Autodesk Inventor part; units mm, degrees
ref_plane "YZ Plane" through (0, 0, 0) normal (1, 0, 0) x (0, 1, 0)
ref_plane "XZ Plane" through (0, 0, 0) normal (0, 1, 0) x (-1, 0, 0)
ref_plane "XY Plane" through (0, 0, 0) normal (0, 0, 1) x (1, 0, 0)
sketch "Sketch7" plane through (0, 0, 0) normal (0, 0, 1) x (1, 0, 0)
  line L0 (0, 21.209) -> (11.3919, 21.209)
  line L1 (11.3919, 21.209) -> (11.3919, 21.209)
  line L2 (11.3919, 21.209) -> (23.6601, 21.209)
  line L3 (23.6601, 21.209) -> (23.6601, 21.209)
  line L4 (23.6601, 21.209) -> (35.052, 21.209)
  line L5 (35.052, 21.209) -> (35.052, 17.526)
  line L6 (0, 17.526) -> (0, 21.209)
  line L7 (0, 17.526) -> (35.052, 17.526)
  line L8 (-6.2642, 17.526) -> (48.9647, 17.526)
  point P0 (0, 0)
  dimension "d57" = 17.526
  dimension "d58" = 7.366
  dimension "d59" = 35.052
  dimension "d60" = 12.2682
  dimension "d128" = 3.683
revolve "Revolution3" add sketch "Sketch7" angle 360 about axis through (-6.2642, 17.526, 0) along (1, 0, 0)
ref_plane "Work Plane3" through (17.526, 17.526, 0) normal (-1, 0, 0) x (0, 0, 1)
sketch "Sketch8" plane through (17.526, 17.526, 0) normal (-1, 0, 0) x (0, 0, 1)
  line L0 (-4.064, 4.064) -> (4.064, 4.064)
  line L1 (4.064, 4.064) -> (4.064, -4.064)
  line L2 (4.064, -4.064) -> (-4.064, -4.064)
  line L3 (-4.064, -4.064) -> (-4.064, 4.064)
  circle A0 centre (0, 0) radius 1.3335
  circle A1 centre (0, 0) radius 3.683
  dimension "d119" = 8.128
  dimension "d121" = 8.128
  dimension "d129" = 4.064
  dimension "d130" = 4.064
extrude "Extrusion5" add sketch "Sketch8" against normal mid plane 12.2936 contours L0 L1 L2 L3 | A1
sketch "Sketch9" plane through (0, 0, 0) normal (0, 0, 1) x (1, 0, 0)
  line L0 (17.526, 15.4328) -> (17.526, -3.476)
  line L1 (11.3792, 13.462) -> (23.6728, 13.462)
  line L2 (17.526, 13.462) -> (21.2458, 13.462)
  line L3 (21.2458, 13.462) -> (21.2458, 9.9568)
  line L4 (21.2458, 9.9568) -> (21.209, 9.9568)
  line L5 (21.209, 9.9568) -> (21.209, 0)
  line L6 (21.209, 0) -> (17.526, 0)
  line L7 (17.526, 0) -> (17.526, 13.462)
  point P0 (0, 0)
  dimension "d65" = 17.526
  dimension "d66" = 7.366
  dimension "d67" = 7.4397
  dimension "d68" = 3.5052
revolve "Revolution4" add sketch "Sketch9" angle 360 about axis through (17.526, 15.4328, 0) along (0, -1, 0)
sketch "Sketch10" plane through (17.526, 9.9568, 0) normal (0, -1, 0) x (1, 0, 0)
  circle A0 centre (0, 0) radius 3.7198
  line L0 (-5.5778, 4.064) -> (5.5778, 4.064)
  line L1 (5.5778, 4.064) -> (5.5778, -4.064)
  line L2 (5.5778, -4.064) -> (-5.5778, -4.064)
  line L3 (-5.5778, -4.064) -> (-5.5778, 4.064)
  line L4 (-6.1468, 4.064) -> (6.1468, 4.064)
  line L5 (-6.1468, -4.064) -> (6.1468, -4.064)
  line L6 (-17.526, -3.683) -> (-17.526, 3.683)
  line L7 (17.526, -3.683) -> (17.526, 3.683)
  dimension "d122" = 11.9482
  dimension "d123" = 11.9482
extrude "Extrusion6" add sketch "Sketch10" against normal up to surface (3.5052 mm away)
sketch "Sketch11" plane through (0, 0, 0) normal (0, 0, 1) x (1, 0, 0)
  line L0 (-6.2642, 17.526) -> (48.9647, 17.526)
  line L1 (0, 21.209) -> (11.3792, 21.209)
  line L2 (8.128, 21.209) -> (8.128, 21.4122)
  line L3 (8.128, 21.209) -> (7.9248, 21.209)
  line L4 (7.9248, 21.209) -> (8.128, 21.4122)
  line L5 (23.6728, 21.59) -> (23.6728, 13.462)
  line L6 (3.81, 21.209) -> (3.81, 21.4122)
  line L7 (3.81, 21.209) -> (3.6068, 21.209)
  line L8 (3.6068, 21.209) -> (3.81, 21.4122)
  line L9 (17.526, 15.4328) -> (17.526, -3.476)
  line L10 (26.924, 21.209) -> (26.924, 21.4122)
  line L11 (26.924, 21.209) -> (27.1272, 21.209)
  line L12 (27.1272, 21.209) -> (26.924, 21.4122)
  line L13 (31.242, 21.209) -> (31.242, 21.4122)
  line L14 (31.242, 21.209) -> (31.4452, 21.209)
  line L15 (31.4452, 21.209) -> (31.242, 21.4122)
  line L16 (0, 13.843) -> (0, 21.209)
  dimension "d75" = 45
  dimension "d114" = 0.2032
  dimension "d115" = 3.81
  dimension "d116" = 4.318
revolve "Revolution5" add sketch "Sketch11" angle 360 about axis through (-6.2642, 17.526, 0) along (1, 0, 0)
sketch "Sketch12" plane through (0, 0, 0) normal (0, 0, 1) x (1, 0, 0)
  line L0 (13.843, 8.4328) -> (13.843, 8.636)
  line L1 (13.843, 8.4328) -> (13.6398, 8.636)
  line L2 (13.6398, 8.636) -> (13.843, 8.636)
  line L3 (17.526, 15.4328) -> (17.526, -3.476)
  line L4 (13.843, 9.9568) -> (13.843, 0)
  line L5 (11.322, 7.2263) -> (14.078, 7.2263)
  line L6 (13.843, 4.1148) -> (13.843, 4.318)
  line L7 (13.843, 4.1148) -> (13.6398, 4.318)
  line L8 (13.6398, 4.318) -> (13.843, 4.318)
  line L9 (13.843, 0) -> (21.209, 0)
  dimension "d89" = 45
  dimension "d90" = 45
  dimension "d124" = 0.2032
  dimension "d125" = 4.318
  dimension "d126" = 4.318
revolve "Revolution6" add sketch "Sketch12" angle 360 about axis through (17.526, 15.4328, 0) along (0, -1, 0)
hole "Hole3" at (35.052, 17.526, 0) direction (-1, 0, 0) diameter 4.7498 end through all
hole "Hole4" at (17.526, 0, 0) direction (0, 1, 0) diameter 4.7498 depth 17.526 tip angle 118
chamfer "Chamfer3" distance 0.3505 angle 30 1 edges at (0, 13.843, 0) measured on face at (1.2023, 21.1613, -0.5908)
chamfer "Chamfer4" distance 0.3505 angle 30 1 edges at (35.052, 13.843, 0) measured on face at (32.6475, 21.1613, -0.5908)
chamfer "Chamfer5" distance 0.3505 angle 30 1 edges at (13.843, 0, 0) measured on face at (21.1971, 2.7432, 0.2964)
fillet "Fillet1" radius 0.5258 2 edges at (11.9482, 13.462, 0) (23.1038, 13.462, 0)
equation "\"d58\" = D1"
equation "\"d59\" = L"
equation "\"d60\" = 0.35 * L"
equation "\"d128\" = 0.5 * D1"
equation "\"d119\" = W1"
equation "\"d121\" = W1"
equation "\"d129\" = 0.5 * W1"
equation "\"d130\" = 0.5 * W1"
equation "\"d63\" = L - 2 * L3"
equation "\"d66\" = D1"
equation "\"d67\" = 1.01 * D1"
equation "\"d68\" = 0.285714 * d60"
equation "\"d122\" = 1.05 * L3"
equation "\"d123\" = 1.05 * L3"
equation "\"d70\" = d60"
equation "\"d114\" = D2"
equation "\"d115\" = L1"
equation "\"d116\" = L2"
equation "\"d124\" = D2"
equation "\"d125\" = L2"
equation "\"d126\" = L2"
equation "\"d95\" = D"
equation "\"d104\" = D"
equation "\"d109\" = M"
equation "\"d111\" = 0.01 * L"
equation "\"d112\" = 0.01 * L"
equation "\"d131\" = 0.01 * L"
equation "\"d132\" = 0.01 * L"
equation "\"d134\" = 0.01 * L"
equation "\"d135\" = 0.01 * L"
equation "\"d127\" = 0.015 * L"
equation "\"L\" = 35.052"
equation "\"M\" = 17.526"
equation "\"D\" = 4.7498"
equation "\"d61\" = 1.75 * D"
equation "\"d84\" = 25.4"
equation "\"d85\" = 1.5748"
equation "\"L1\" = 3.81"
equation "\"L2\" = 4.318"
equation "\"L3\" = 11.3792"
equation "\"D1\" = 7.366"
equation "\"D2\" = 0.2032"
equation "\"W1\" = 8.128"
equation "\"d117\" = -0.5 * L"
properties part number "Tubo en T de unión 224 de Parker 224-6" material "Latón, amarillo claro"
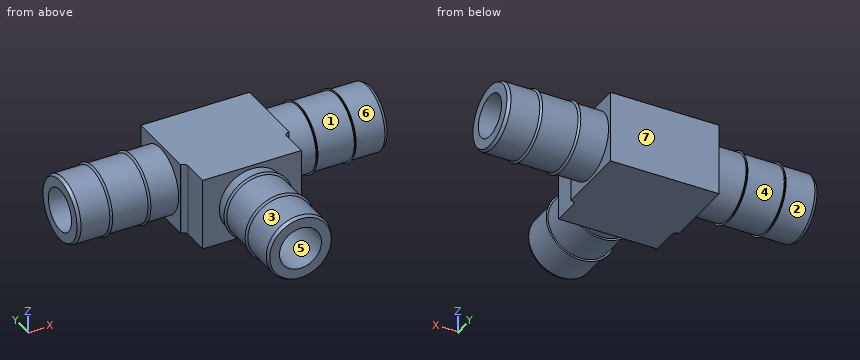
The listing builds one solid part. Answer for the finished solid, in the listing's coordinates (mm). Face numbers are marked on the shaded views. A direction names the side the tool comes from. Coordinates: 2 decimals unless noted, no trailing zeros. Write each loop counter-clockwise with the first axis right and the second up, starting at its lowest first coordinate (ties: lowest second). Pieces come first, ordered by that corner, then holes. Notation, with made-up numbers: M 10.25,-35.75 L 27.25,-35.75 A32 ccw 27.25,3.25 Z; hole C -8,84.5 d2. An arc over 180 degrees is marked long. Use a Markdown table: item, result. Add a question column.
1. Section B-B (z = 0) is taken. Count the separate pieces of the cut face and the enclosed holes in it, plus the area to 3 significant figures.
2. For a pull along X with two mould halves and no side action, classify the marked faces 1, 2 and 3 as +X half, -X half, draft (parallel to the pull), parting line (faces both ways), or undercut.
3. Given P1, Ø1.5, axis at x = 28.5, z = 3, coming from the +Y side; P2, Ø3, axis at y = 16.5, z = -1, coming from the +X side; P3, Ø0.9, axis at y = 12, z = 0, coming from the -X side; P4, Ø1.5, axis at y = 12, z = 0.5, coming from the +X side, each flat-ended and moving along its own axis, determine where each tip first touches the part or whether it passes through.
4. Section A-A (x = 26) is taken. Give the vertices of the cut face in (y, z), plus the area to 3 significant figures.
5. Which of the six approach directions +Z, -Z, +X, -X, +Y, -Y give full straight-line access (tool end or side, diameter ignored) to the marked faces 4, 5, 6 and 7?
6. Straight lines are drawn through the part: line 1 along X through (y, z) = (6.25, 0); line 2 along X through (y, z) = (14.25, 0); line 3 along Z through (x, y) = (22.5, 17.5). For each, find the intervals that lie inside material, in ascending order. Write a range as [from, to].
Data:
| question | item | result |
|---|---|---|
| 1 | separate pieces | 3 |
| 1 | enclosed holes | 0 |
| 1 | area | 142 mm2 |
| 2 | face 1 | undercut |
| 2 | face 2 | draft |
| 2 | face 3 | parting line |
| 3 | P1 | stops at y = 20.44 |
| 3 | P2 | stops at x = 35.05 |
| 3 | P3 | stops at x = 11.95 |
| 3 | P4 | stops at x = 23.1 |
| 4 | outline | C 17.53,0 d7.37; hole C 17.53,0 d4.75 |
| 4 | area | 24.9 mm2 |
| 5 | face 4 | none |
| 5 | face 5 | -Y |
| 5 | face 6 | +X |
| 5 | face 7 | +Z, -Z, +X, -X, +Y |
| 6 | line 1 | x = [13.84, 15.15], [19.9, 21.21] |
| 6 | line 2 | x = [0, 15.15], [19.9, 35.05] |
| 6 | line 3 | z = [-4.06, -2.37], [2.37, 4.06] |
